Can you work these out from the model? Positions are in its coordinate system, mm. Face numbers are marked on the shaded views. A direction names the side the tool comes from. Coordinates: 2 decimals unless noted, no trailing zeros. Order: outer loops, then holes, each group sorted by start corner. A loop starts at its lowest first (then second) coordinate and runs counter-clockwise, first axis right, second up.
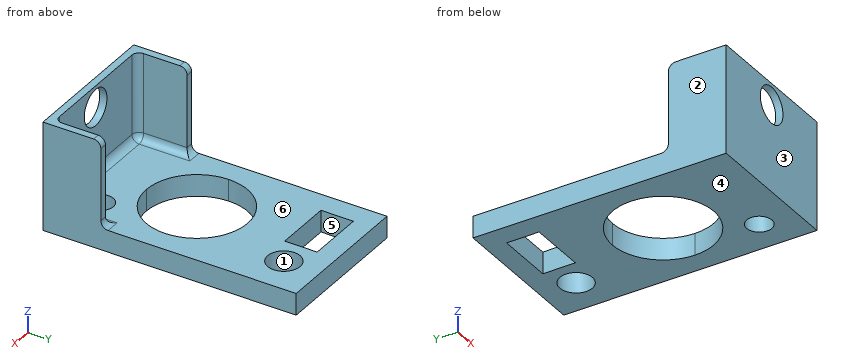
```python
from build123d import *

# Parameters (mm, degrees)
SKETCH1_7_W         = 18
SKETCH1_7_H         = 33
SKETCH1_7_R         = 2.25
SKETCH1_7_R_2       = 1.75
SKETCH1_7_W_2       = 14
SKETCH1_7_H_2       = 14
SKETCH1_7_W_3       = 8
SKETCH1_7_H_3       = 4.5
SKETCH1_7_H_4       = 1
BOSS_EXTRUDE2_DEPTH = 3
SKETCH1_8_W         = 18
SKETCH1_8_H         = 1
BOSS_EXTRUDE3_DEPTH = 12
SKETCH2_R           = 2.5
CUT_EXTRUDE1_DEPTH  = 43.05948169
FILLET1_R           = 1


with BuildPart() as part:
    # Sketch1_7 → Boss-Extrude2 (new body)
    # profile 1 of 9: a face of its own
    with BuildSketch(Plane.XY):
        with Locations((10, 37.5)):
            Rectangle(SKETCH1_7_W, SKETCH1_7_H)
        with Locations((14.75, 50)):
            Circle(SKETCH1_7_R, mode=Mode.SUBTRACT)
        with Locations((15.25, 25)):
            Circle(SKETCH1_7_R_2, mode=Mode.SUBTRACT)
        with Locations((10, 35)):
            Rectangle(SKETCH1_7_W_2, SKETCH1_7_H_2, mode=Mode.SUBTRACT)
        with Locations((7, 50)):
            Rectangle(SKETCH1_7_W_3, SKETCH1_7_H_3, mode=Mode.SUBTRACT)
    # profile 2 of 9: a face of its own
    with BuildSketch(Plane.XY):
        Polygon((0, 28), (0, 20), (1, 20), (1, 21), (1, 28), align=None)
    # profile 3 of 9: a face of its own
    with BuildSketch(Plane.XY):
        with Locations((10, 20.5)):
            Rectangle(SKETCH1_7_W, SKETCH1_7_H_4)
    # profile 4 of 9: a face of its own
    with BuildSketch(Plane.XY):
        Polygon((19, 21), (19, 20), (20, 20), (20, 28), (19, 28), align=None)
    # profile 5 of 9: a face of its own
    with BuildSketch(Plane.XY):
        Polygon((0, 55), (0, 28), (1, 28), (1, 54), (19, 54), (19, 28), (20, 28), (20, 55), align=None)
    # profile 6 of 9: a face of its own
    with BuildSketch(Plane.XY):
        with BuildLine():
            ThreePointArc((10, 28), (5.050252532, 30.050252532), (3, 35))
            Line((3, 35), (3, 28))
            Line((3, 28), (10, 28))
        make_face()
    # profile 7 of 9: a face of its own
    with BuildSketch(Plane.XY):
        with BuildLine():
            ThreePointArc((3, 35), (5.050252532, 39.949747468), (10, 42))
            Line((10, 42), (3, 42))
            Line((3, 42), (3, 35))
        make_face()
    # profile 8 of 9: a face of its own
    with BuildSketch(Plane.XY):
        with BuildLine():
            Line((17, 35), (17, 42))
            Line((17, 42), (10, 42))
            ThreePointArc((10, 42), (14.949747468, 39.949747468), (17, 35))
        make_face()
    # profile 9 of 9: a face of its own
    with BuildSketch(Plane.XY):
        with BuildLine():
            Line((17, 28), (17, 35))
            ThreePointArc((17, 35), (14.949747468, 30.050252532), (10, 28))
            Line((10, 28), (17, 28))
        make_face()
    extrude(amount=-BOSS_EXTRUDE2_DEPTH)

    # Sketch1_8 → Boss-Extrude3 (add)
    with BuildSketch(Plane.XY):
        Polygon((19, 21), (19, 20), (20, 20), (20, 28), (19, 28), align=None)
        with Locations((10, 20.5)):
            Rectangle(SKETCH1_8_W, SKETCH1_8_H)
        Polygon((0, 28), (0, 20), (1, 20), (1, 21), (1, 28), align=None)
    extrude(amount=BOSS_EXTRUDE3_DEPTH)

    # Sketch2 → Cut-Extrude1 (cut, through all)
    with BuildSketch(Plane.XZ.offset(-20)):
        with Locations((10, 9)):
            Circle(SKETCH2_R)
    extrude(amount=-CUT_EXTRUDE1_DEPTH, mode=Mode.SUBTRACT)

    # Fillet1
    fillet1_edges = [part.edges().sort_by_distance(p)[0] for p in [
        (19.5, 28, 12),
        (0.5, 28, 12),
        (1, 24.5, 0),
        (19, 24.5, 0),
        (19, 21, 6),
        (10, 21, 0),
        (1, 21, 6),
        (19.5, 28, 0),
        (0.5, 28, 0),
    ]]
    fillet(fillet1_edges, radius=FILLET1_R)


solid = part.part
```
1. Please list where these lines run through material, in increasing order: probe 1 along Y at (x, z) = (15.25, -1.35); probe 2 along X at (y, z) = (27, 7); probe 3 along Y at (x, z) = (14.75, -0.65).
Completed:
probe 1: y = 20 to 23.25, 26.75 to 30.37, 39.63 to 47.81, 52.19 to 55
probe 2: x = 0 to 1, 19 to 20
probe 3: y = 20 to 23.32, 26.68 to 29.86, 40.14 to 47.75, 52.25 to 55
2. Imagine slicing it at B-B on y = 50. Please give me the cut outline in (x, z).
Completed:
outline: (0, -3) - (3, -3) - (3, 0) - (0, 0) - close; (11, -3) - (12.5, -3) - (12.5, 0) - (11, 0) - close; (17, -3) - (20, -3) - (20, 0) - (17, 0) - close
3. I'm going to push flat-ended pins straight in: pin 1 (6 mm diameter, centred on x = 11.5, y = 43, fed in from +Z); pin 2 (2 mm diameter, centred on x = 15.25, y = 25, fed in from +Z). Where does each tip first touch, or does it pass through?
Completed:
pin 1: stops at z = 0
pin 2: passes through
4. Imagine slicing it at C-C on y = 25. Please give me the cut outline in (x, z).
Completed:
outline: (0, -3) - (13.5, -3) - (13.5, 0) - (2, 0) arc R1 cw to (1, 1) - (1, 12) - (0, 12) - close; (17, -3) - (20, -3) - (20, 12) - (19, 12) - (19, 1) arc R1 cw to (18, 0) - (17, 0) - close
5. On a 3-axis mill with a long thin cutter (end or side, diameter ignored), from which of +Z, -Z, +X, -X, +Y, -Y can I reach the whole of each face in a straight line? I mean the marked faces 4, 5 and 6. Say none if no direction works.
Completed:
face 4: -Z, +X, -X, +Y, -Y
face 5: +Z, -Z
face 6: +Z, +Y
6. Thinking about a two-plate mould opening in X: for the marked faces 1, 2 and 3, which applies, pulls with the +X half, pulls with the -X half, needs draft (parallel to the pull), parting line crosses it, or undercut?
Completed:
face 1: undercut
face 2: pulls with the -X half
face 3: needs draft
7. Imagine slicing it at A-A on z = 9. Please give me the cut outline in (x, y).
Completed:
outline: (0, 20) - (7.5, 20) - (7.5, 21) - (2, 21) arc R1 cw to (1, 22) - (1, 28) - (0, 28) - close; (12.5, 20) - (20, 20) - (20, 28) - (19, 28) - (19, 22) arc R1 cw to (18, 21) - (12.5, 21) - close
8. Imagine slicing it at D-D on x = 9. Please give me the cut outline in (y, z).
Completed:
outline: (20, -3) - (28.07, -3) - (28.07, 0) - (22, 0) arc R1 cw to (21, 1) - (21, 6.71) - (20, 6.71) - close; (20, 11.29) - (21, 11.29) - (21, 12) - (20, 12) - close; (41.93, -3) - (47.75, -3) - (47.75, 0) - (41.93, 0) - close; (52.25, -3) - (55, -3) - (55, 0) - (52.25, 0) - close
